Geometry check sheet. Reference: drawing and pictorial views, mm from the part's lowest x, y, z. A direction names the side the tool comes from. Give positions to 0.01 mm unless a question says otherwise; leave off trailing zeros. Write each loop counter-clockwise with the first axis right and the second up, starting at its lowest first coordinate (ties: lowest second). Pieces come first, ordered by that corner, then holes. Notation, with made-up numbers: M 51.25,21.5 L 62.25,21.5 A5 ccw 62.25,29.5 Z; hole C 88.25,46.25 d2. An arc over 180 degrees is marked long. One line per item, written item: value. Start each with the question number.
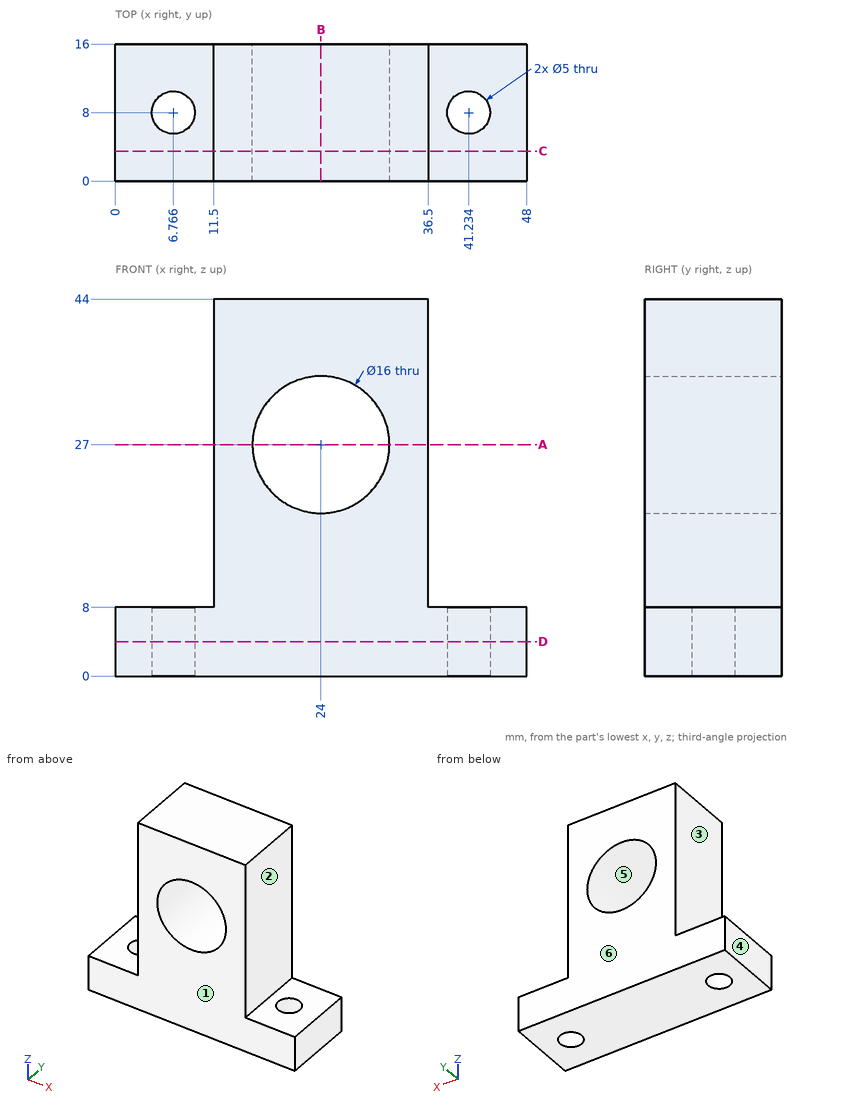
1) Material ranges on L1, parallel to Z at x = 24, y = 6; L2, parallel to X at y = 9.25, z = 9.5; L3, parallel to Z at x = 43.5, y = 3.5, recorded low to high. Write a range as from..to.
2) Cross-section at C-C (y = 3.5). Record the boundary of the cut face in (x, z), plus the area to 3 significant figures.
3) Gauge pin test, flat ends, axial feed: pin 1 (6 mm diameter, centred on x = 42.5, y = 8.5, fed in from +Z); pin 2 (3 mm diameter, centred on y = 5, z = 11, fed in from -X); pin 3 (6 mm diameter, centred on y = 4.5, z = 36.5, fed in from +X); pin 4 (3 mm diameter, centred on x = 41.23, y = 8, fed in from -Z). Record the tip position at first contact, or that the pin passes through.
4) Cross-section at B-B (x = 24). Record the boundary of the cut face in (y, z).
5) Draft check along X on the marked faces 4, 5 and 6. Enter one of: released by +X, released by -X, zero draft, split by the parting line, or undercut.
6) Tool access check on the marked faces 1, 2 and 3. Record the directions out of +Z, -Z, +X, -X, +Y, -Y that give a thin tool (end or side, any length) a straight path to the whole face; none if there is none.
7) Cross-section at D-D (z = 4). Record the boundary of the cut face in (x, y).
8) Cross-section at A-A (z = 27). Record the boundary of the cut face in (x, y), plus the area to 3 significant figures.
Data:
1. L1: z = 0..19, 35..44
1. L2: x = 11.5..36.5
1. L3: z = 0..8
2. outline: M 0,0 L 48,0 L 48,8 L 36.5,8 L 36.5,44 L 11.5,44 L 11.5,8 L 0,8 Z; hole C 24,27 d16
2. area: 1,080 mm2
3. pin 1: stops at z = 8
3. pin 2: stops at x = 11.5
3. pin 3: stops at x = 36.5
3. pin 4: passes through
4. outline: M 0,0 L 16,0 L 16,19 L 0,19 Z; M 0,35 L 16,35 L 16,44 L 0,44 Z
5. face 4: released by -X
5. face 5: undercut
5. face 6: zero draft
6. face 1: +Z, -Z, +X, -X, -Y
6. face 2: +Z, +X, +Y, -Y
6. face 3: +Z, -X, +Y, -Y
7. outline: M 0,0 L 48,0 L 48,16 L 0,16 Z; hole C 6.77,8 d5; hole C 41.23,8 d5
8. outline: M 11.5,0 L 16,0 L 16,16 L 11.5,16 Z; M 32,0 L 36.5,0 L 36.5,16 L 32,16 Z
8. area: 144 mm2
